Geometry check sheet. Reference: the model listing, model coordinates, mm. A direction names the side the tool comes from. Coordinates: 2 decimals unless noted, no trailing zeros. Order: outer loops, then holes, each group sorted by start corner. A loop starts at its lowest first (then second) coordinate and runs counter-clockwise, first axis right, second up. Notation, with made-up numbers: M -26,52.5 L 14,52.5 A15 cw 14,70.5 Z; hole C 43,52.5 d10. An arc over 180 degrees is marked long. One line per item, written item: value. Start each with the question number.
1) Sectioned sample at D-D, the plane x = -60. Enter the section's corners in (y, z).
2) Sectioned sample at C-C, the plane y = 51.5. Enter the section's corners in (x, z), then the cut area to 3 significant figures.
3) Access from +Z, -Z, +X, -X, +Y, -Y to the whole of each face (thin tool, end or side, straight path). Record for faces 1 (the flat face through (22, 28, 0)), 2 (the flat face through (-12.5, 5, 46)), 3 (the flat face through (46, 5, 12.5)), 4 (the flat face through (60, 6, -2)), 5 (the flat face through (-46, 5, -12.5)).
4) Sectioned sample at A-A, the plane x = 62.5. Enter the section's corners in (y, z), then the cut area to 3 significant figures.
5) Sectioned sample at B-B, the plane z = 0. State how many separate pieces and enclosed holes the cut face has, then the cut area to 3 significant figures.
6) Thickness scan on L1, parallel to X at y = 36, z = 0; L2, parallel to Y at x = 0, z = 61.5; L3, parallel to Z at x = -57, y = 6. Record the ranges inside material, lowest first. Write a range as from..to.
7) Go/stop test with flat-tipped pins: P1, Ø0.6, axis at x = 61, y = 11, coming from the -Z side; P2, Ø4.5, axis at y = 3.5, z = 51, coming from the -X side; P3, Ø10, axis at y = 3.5, z = -35, coming from the +X side. Record where each tip stops, or that it passes through.
8) Draft check along Y on faces 6 (the flat face through (45, 6, -2)), 7 (the cylindrical face through (-70, 5, 0)), 8 (the flat face through (22, 19, -7.5)). Enter one of: pulls with the +Y half, pulls with the -Y half, needs draft (parallel to the pull), parting line crosses it, or undercut.
```python
from build123d import *

# Parameters (mm, degrees)
BOSS_EXTRUDE1_DEPTH = 10
SKETCH2_R           = 25
SKETCH2_R_2         = 21
BOSS_EXTRUDE2_DEPTH = 60
SKETCH3_W           = 15
SKETCH3_H           = 18
CUT_EXTRUDE1_DEPTH  = 10
SKETCH4_W           = 25
SKETCH4_H           = 12.7
BOSS_EXTRUDE3_DEPTH = 2
SKETCH5_R           = 2.75
CUT_EXTRUDE2_DEPTH  = 115.734476074
SKETCH6_R           = 5
CUT_EXTRUDE3_DEPTH  = 6
FILLET1_R           = 1


with BuildPart() as part:
    # Sketch1 → Boss-Extrude1 (new body)
    with BuildSketch(Plane(origin=(0, 0, 0), x_dir=(1, 0, 0), z_dir=(0, 1, 0))):
        with BuildLine():
            Line((-68.87488657, 12.5), (-21.650635095, 12.5))
            ThreePointArc((-21.650635095, 12.5), (-17.67766953, 17.67766953), (-12.5, 21.650635095))
            Line((-12.5, 21.650635095), (-12.5, 68.87488657))
            ThreePointArc((-12.5, 68.87488657), (0, 70), (12.5, 68.87488657))
            Line((12.5, 68.87488657), (12.5, 21.650635095))
            ThreePointArc((12.5, 21.650635095), (17.67766953, 17.67766953), (21.650635095, 12.5))
            Line((21.650635095, 12.5), (68.87488657, 12.5))
            ThreePointArc((68.87488657, 12.5), (70, 0), (68.87488657, -12.5))
            Line((68.87488657, -12.5), (21.650635095, -12.5))
            ThreePointArc((21.650635095, -12.5), (17.67766953, -17.67766953), (12.5, -21.650635095))
            Line((12.5, -21.650635095), (12.5, -68.87488657))
            ThreePointArc((12.5, -68.87488657), (0, -70), (-12.5, -68.87488657))
            Line((-12.5, -68.87488657), (-12.5, -21.650635095))
            ThreePointArc((-12.5, -21.650635095), (-17.67766953, -17.67766953), (-21.650635095, -12.5))
            Line((-21.650635095, -12.5), (-68.87488657, -12.5))
            ThreePointArc((-68.87488657, -12.5), (-70, 0), (-68.87488657, 12.5))
        make_face()
    extrude(amount=BOSS_EXTRUDE1_DEPTH)

    # Sketch2 → Boss-Extrude2 (add)
    with BuildSketch(Plane(origin=(0, 10, 0), x_dir=(1, 0, 0), z_dir=(0, 1, 0))):
        with Locations(Location((0, 0, 0), (0, 0, 120))):
            Circle(SKETCH2_R)
        with Locations(Location((0, 0, 0), (0, 0, 270))):
            Circle(SKETCH2_R_2, mode=Mode.SUBTRACT)
    extrude(amount=BOSS_EXTRUDE2_DEPTH)

    # Sketch3 → Cut-Extrude1 (cut)
    with BuildSketch(Plane(origin=(25, 0, 0), x_dir=(0, 0, -1), z_dir=(1, 0, 0))):
        with Locations((0, 19)):
            Rectangle(SKETCH3_W, SKETCH3_H)
    extrude(amount=-CUT_EXTRUDE1_DEPTH, mode=Mode.SUBTRACT)

    # Sketch4 → Boss-Extrude3 (add)
    with BuildSketch(Plane(origin=(0, 10, 0), x_dir=(1, 0, 0), z_dir=(0, 1, 0))):
        with Locations((55, 0)):
            Rectangle(SKETCH4_W, SKETCH4_H)
    extrude(amount=BOSS_EXTRUDE3_DEPTH)

    # Sketch5 → Cut-Extrude2 (cut, through all)
    with BuildSketch(Plane(origin=(0, 12, 0), x_dir=(1, 0, 0), z_dir=(0, 1, 0))):
        with Locations(Location((47.5, 0, 0), (0, 0, 270))):
            Circle(SKETCH5_R)
        with Locations(Location((62.5, 0, 0), (0, 0, 90))):
            Circle(SKETCH5_R)
    extrude(amount=-CUT_EXTRUDE2_DEPTH, mode=Mode.SUBTRACT)

    # Sketch6 → Cut-Extrude3 (cut)
    with BuildSketch(Plane.XZ):
        with Locations(Location((47.5, 0, 0), (0, 0, 270))):
            Circle(SKETCH6_R)
        with Locations(Location((62.5, 0, 0), (0, 0, 270))):
            Circle(SKETCH6_R)
    extrude(amount=-CUT_EXTRUDE3_DEPTH, mode=Mode.SUBTRACT)

    # Fillet1
    fillet1_edges = [part.edges().sort_by_distance(p)[0] for p in [
        (47.5, 0, 5),
        (62.5, 0, 5),
        (-45.262760832, 0, -12.5),
        (-17.67766953, 0, -17.67766953),
        (-12.5, 0, -45.262760832),
        (0, 0, -70),
        (12.5, 0, -45.262760832),
        (17.67766953, 0, -17.67766953),
        (45.262760832, 0, -12.5),
        (70, 0, 0),
        (45.262760832, 0, 12.5),
        (17.67766953, 0, 17.67766953),
        (12.5, 0, 45.262760832),
        (0, 0, 70),
        (-12.5, 0, 45.262760832),
        (-17.67766953, 0, 17.67766953),
        (-45.262760832, 0, 12.5),
        (-70, 0, 0),
        (0, 70, -21),
    ]]
    fillet(fillet1_edges, radius=FILLET1_R)


solid = part.part
```
Final values:
1. outline: M 0,-11.5 A1 ccw 1,-12.5 L 10,-12.5 L 10,12.5 L 1,12.5 A1 ccw 0,11.5 Z
2. outline: C 0,0 d50; hole C 0,0 d42
2. area: 578 mm^2
3. face 1: +X
3. face 2: +Z, -X, +Y, -Y
3. face 3: +Z, +X, +Y, -Y
3. face 4: -Y
3. face 5: -Z, -X, +Y, -Y
4. outline: M 0,-11.5 A1 ccw 1,-12.5 L 10,-12.5 L 10,-6.35 L 12,-6.35 L 12,-2.75 L 6,-2.75 L 6,-5 L 1,-5 A1 ccw 0,-6 Z; M 0,6 A1 ccw 1,5 L 6,5 L 6,2.75 L 12,2.75 L 12,6.35 L 10,6.35 L 10,12.5 L 1,12.5 A1 ccw 0,11.5 Z
4. area: 182 mm^2
5. separate pieces: 4
5. enclosed holes: 0
5. area: 1,670 mm^2
6. L1: x = -25..-21, 21..25
6. L2: y = 0..10
6. L3: z = -12.5..12.5
7. P1: stops at z = -6.35
7. P2: stops at x = -12.5
7. P3: stops at x = 12.5
8. face 6: pulls with the -Y half
8. face 7: needs draft
8. face 8: undercut
